Could you check a few things on this model? Use its own coordinates, in mm. A direction names the side the tool comes from. Round coordinates to 2 decimals unless told otherwise and drop trailing zeros. Loops run counter-clockwise (first coordinate to the right, second up) from the corner with the lowest first, then second, coordinate; pieces in that order, holes last. Notation, with made-up numbers: (-18, 49) -> (37, 49) arc R18 cw to (37, 61) -> close; hole circle Ø4 at (-37, 65.5). An arc over 180 degrees is marked (long way). One line per item, written item: value.
from build123d import *

# Parameters (mm, degrees)
PAD097_DEPTH        = 10
SKETCH351_W         = 3
SKETCH351_H         = 2.4
PAD098_DEPTH        = 3
HOLE_D              = 5.5
HOLE_CBORE_D        = 10
HOLE_CBORE_DEPTH    = 5.4
HOLE041_D           = 4.5
HOLE041_DEPTH       = 7
HOLE041_CBORE_D     = 5.6
HOLE041_CBORE_DEPTH = 4
HOLE041_TIPS_R      = 2.25
CHAMFER006_SIZE     = 0.4


with BuildPart() as part:
    # Sketch350 → Pad097 (new body, symmetric)
    with BuildSketch(Plane.XY):
        Polygon((92, 73), (103, 73), (103, 46.573101), (98.597712, 46.573101), (92, 58.23869), align=None)
    extrude(amount=PAD097_DEPTH, both=True)

    # Sketch351 → Pad098 (join, symmetric)
    with BuildSketch(Plane.XY):
        Polygon((103, 46.573101), (106, 46.573101), (106, 57.5), (103, 60.5), align=None)
        with Locations((104.5, 71.8)):
            Rectangle(SKETCH351_W, SKETCH351_H)
    extrude(amount=PAD098_DEPTH, both=True)

    # Hole (through all)
    with Locations(Plane(origin=(92, 0, 0), x_dir=(0, -1, 0), z_dir=(-1, 0, 0))):
        with Locations((-65.5, 0)):
            CounterBoreHole(HOLE_D / 2, HOLE_CBORE_D / 2, HOLE_CBORE_DEPTH)

    # Hole041
    with Locations(Plane(origin=(94.659391, 53.536551, 0), x_dir=(0.49229, -0.870431, 0), z_dir=(-0.870431, -0.49229, 0))):
        with Locations((0, 0)):
            CounterBoreHole(HOLE041_D / 2, HOLE041_CBORE_D / 2, HOLE041_CBORE_DEPTH, depth=HOLE041_DEPTH)

    # Hole041 tips → Hole041 tip 1 section 0
    with BuildSketch(Plane(origin=(100.752409, 56.982581, 0), x_dir=(0.49229, -0.870431, 0), z_dir=(-0.870431, -0.49229, 0)), mode=Mode.PRIVATE) as hole041_tip_1_s0:
        Circle(HOLE041_TIPS_R)
    loft([hole041_tip_1_s0.sketch, Vertex(101.929177, 57.648126, 0)], mode=Mode.SUBTRACT)

    # Chamfer006
    chamfer006_edges = [part.edges().sort_by_distance(p)[0] for p in [
        (97.5, 73, 10),
        (103, 59.786551, 10),
        (100.798856, 46.573101, 10),
        (95.298856, 52.405895, 10),
        (92, 65.619345, 10),
        (98.597712, 46.573101, 0),
        (97.5, 73, -10),
        (103, 59.786551, -10),
        (100.798856, 46.573101, -10),
        (95.298856, 52.405895, -10),
        (92, 65.619345, -10),
        (92, 73, 0),
        (103, 46.573101, 6.5),
        (104.5, 73, 3),
        (104.5, 73, -3),
    ]]
    chamfer(chamfer006_edges, length=CHAMFER006_SIZE)


with BuildPart() as part_1:
    # Body022073 placement: moved
    add(part.part.moved(Location((0, 0, -132))))


solid = part_1.part
(1) If we section it at B-B, the plane x = 104.75: Please give me the cut outline in (y, z).
Recorded:
outline: (46.57, -135) -> (58.75, -135) -> (58.75, -129) -> (46.57, -129) -> close; (70.6, -135) -> (72.6, -135) -> (73, -134.6) -> (73, -129.4) -> (72.6, -129) -> (70.6, -129) -> close
(2) If we section it at C-C, the plane z = -125.25: Please give me the cut outline in (x, y), then the cut area to 3 significant figures.
Recorded:
outline: (92, 58.24) -> (98.4, 46.92) -> (99, 46.57) -> (102.6, 46.57) -> (103, 46.97) -> (103, 73) -> (92.4, 73) -> (92, 72.6) -> close
area: 252 mm²
(3) Thinking about a two-plate mould opening in Y: for faces 5 (the face through (98, 60, -122)), 6 (the face through (95.42, 52.6, -122.2)), 7 (the face through (97.69, 52.18, -131.16)), which applies, released by +Y, released by -Y, zero draft, split by the parting line, or undercut?
Recorded:
face 5: zero draft
face 6: released by -Y
face 7: undercut
(4) I'm going to push flat-ended pins straight in: pin 1 Ø0.6 at (x, y) = (104, 71.5) entering from +Z; pin 2 Ø9 at (y, z) = (65.5, -132) entering from -X; pin 3 Ø0.9 at (x, y) = (104, 54) entering from -Z. Where does each tip first touch, or does it pass through?
Recorded:
pin 1: z = -129
pin 2: x = 97.4
pin 3: z = -135
(5) For faces 1 (the face through (94.662, 63.193, -136.436)), 2 (the face through (95.42, 52.6, -141.8)), 3 (the face through (104, 54, -135)), 4 (the face through (104.5, 59, -132)), which set-ups out of +Z, -Z, +X, -X, +Y, -Y let a thin tool reach every point of the face, with its end or its side?
Recorded:
face 1: -X
face 2: -Z, -X, -Y
face 3: -Z, +X, +Y, -Y
face 4: +Z, -Z, +X
(6) If I drill on L1, parallel to Z at x = 95.7, y = 65.5; L2, parallel to Z at x = 101.2, y = 65.5; L3, parallel to Y at x = 100.3, z = -132, over which ranges is the centre line in solid material (lowest first)?
Recorded:
L1: -142 to -137, -127 to -122
L2: -142 to -134.75, -129.25 to -122
L3: 46.57 to 54.14, 58.57 to 62.75, 68.25 to 73
(7) If we section it at A-A, the plane y = 65.5: Please give me the cut outline in (x, z).
Recorded:
outline: (92, -141.6) -> (92.4, -142) -> (102.6, -142) -> (103, -141.6) -> (103, -134.75) -> (97.4, -134.75) -> (97.4, -137) -> (92, -137) -> close; (92, -127) -> (97.4, -127) -> (97.4, -129.25) -> (103, -129.25) -> (103, -122.4) -> (102.6, -122) -> (92.4, -122) -> (92, -122.4) -> close
(8) If we section it at D-D, the plane y = 59.25: Please give me the cut outline in (x, z).
Recorded:
outline: (92, -141.6) -> (92.4, -142) -> (102.6, -142) -> (103, -141.6) -> (103, -135) -> (104.25, -135) -> (104.25, -129) -> (103, -129) -> (103, -122.4) -> (102.6, -122) -> (92.4, -122) -> (92, -122.4) -> close
